from build123d import *

# Parameters (mm, degrees)
ESQUISSE1_W        = 48
ESQUISSE1_H        = 22
ESQUISSE1_R        = 2
ESQUISSE1_R_2      = 1.5
BOSS_EXTRU_1_DEPTH = 3
CONG_1_R           = 4


with BuildPart() as part:
    # Esquisse1 → Boss.-Extru.1 (new body)
    with BuildSketch(Plane.XY):
        with Locations((24, -11)):
            Rectangle(ESQUISSE1_W, ESQUISSE1_H)
        with Locations((24, -3.5)):
            Circle(ESQUISSE1_R, mode=Mode.SUBTRACT)
        with Locations((24, -18.5)):
            Circle(ESQUISSE1_R, mode=Mode.SUBTRACT)
        with Locations((4, -3.5)):
            Circle(ESQUISSE1_R_2, mode=Mode.SUBTRACT)
        with Locations((44, -3.5)):
            Circle(ESQUISSE1_R_2, mode=Mode.SUBTRACT)
        with Locations((44, -18.5)):
            Circle(ESQUISSE1_R_2, mode=Mode.SUBTRACT)
        with Locations((4, -18.5)):
            Circle(ESQUISSE1_R_2, mode=Mode.SUBTRACT)
    extrude(amount=BOSS_EXTRU_1_DEPTH)

    # Congé1
    cong_1_edges = [part.edges().sort_by_distance(p)[0] for p in [
        (0, 0, 1.5),
        (48, 0, 1.5),
        (48, -22, 1.5),
        (0, -22, 1.5),
    ]]
    fillet(cong_1_edges, radius=CONG_1_R)


solid = part.part
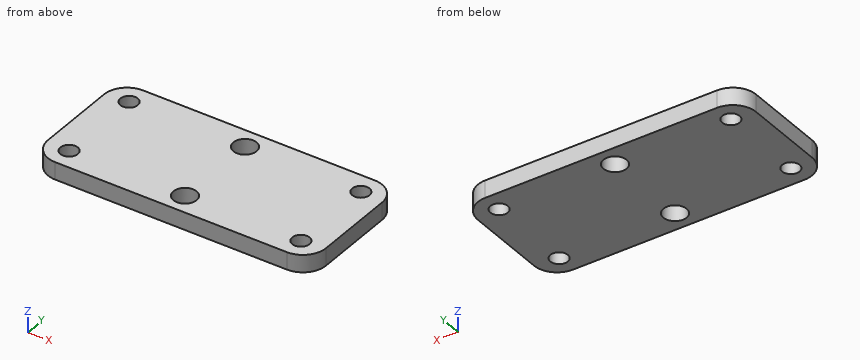
Can you work these out from the model? Positions are in its coordinate system, mm. Coordinates: 2 decimals unless noted, no trailing zeros. Loops run counter-clockwise (first coordinate to the right, second up) from the corner with the lowest first, then second, coordinate; pieces in that order, holes last. Notation, with made-up numbers: (19, -14) - (39, -14) arc R27 ccw to (39, 4) - close; hole circle Ø3 at (-11.5, 39.25). An arc over 180 degrees is marked (long way). Put each result on its own line as item: value. Start each with the question number.
Item 1: For pin 1 (2.5 mm diameter, centred on x = 44, y = -3.5, fed in from -Z), with a flat end and sliding along its axis, tell me the tip position at first contact or that it passes through.
Item 2: Suppose I cut it at D-D (x = 24). Please give me the cut outline in (y, z).
Item 3: Suppose I cut it at A-A (z = 0.55). Please give me the cut outline in (x, y).
Item 4: If I drill on line 1 along Y through (x, z) = (4, 1.1); line 2 along Y through (x, z) = (24, 1.7); line 3 along X through (y, z) = (-19.5, 2.5), over which ranges is the centre line in solid material (lowest first)?
Item 5: Suppose I cut it at C-C (y = -3.5). Please give me the cut outline in (x, z), and give its area (3 significant figures).
Item 6: Suppose I cut it at B-B (x = 43). Please give me the cut outline in (y, z).
Here are the results:
1. pin 1: through
2. outline: (-22, 0) - (-20.5, 0) - (-20.5, 3) - (-22, 3) - close; (-16.5, 0) - (-5.5, 0) - (-5.5, 3) - (-16.5, 3) - close; (-1.5, 0) - (0, 0) - (0, 3) - (-1.5, 3) - close
3. outline: (0, -18) arc R4 ccw to (4, -22) - (44, -22) arc R4 ccw to (48, -18) - (48, -4) arc R4 ccw to (44, 0) - (4, 0) arc R4 ccw to (0, -4) - close; hole circle Ø3 at (4, -18.5); hole circle Ø3 at (4, -3.5); hole circle Ø4 at (24, -18.5); hole circle Ø4 at (24, -3.5); hole circle Ø3 at (44, -18.5); hole circle Ø3 at (44, -3.5)
4. line 1: -22 to -20, -17 to -5, -2 to 0
4. line 2: -22 to -20.5, -16.5 to -5.5, -1.5 to 0
4. line 3: 0.29 to 2.88, 5.12 to 22.27, 25.73 to 42.88, 45.12 to 47.71
5. outline: (0.03, 0) - (2.5, 0) - (2.5, 3) - (0.03, 3) - close; (5.5, 0) - (22, 0) - (22, 3) - (5.5, 3) - close; (26, 0) - (42.5, 0) - (42.5, 3) - (26, 3) - close; (45.5, 0) - (47.97, 0) - (47.97, 3) - (45.5, 3) - close
5. area: 114 mm²
6. outline: (-22, 0) - (-19.62, 0) - (-19.62, 3) - (-22, 3) - close; (-17.38, 0) - (-4.62, 0) - (-4.62, 3) - (-17.38, 3) - close; (-2.38, 0) - (0, 0) - (0, 3) - (-2.38, 3) - close
